Autodesk Inventor part; units mm, degrees
ref_plane "YZ Plane" through (0, 0, 0) normal (1, 0, 0) x (0, 1, 0)
ref_plane "XZ Plane" through (0, 0, 0) normal (0, 1, 0) x (-1, 0, 0)
ref_plane "XY Plane" through (0, 0, 0) normal (0, 0, 1) x (1, 0, 0)
sketch "Sketch1" plane through (0, 0, 0) normal (0, 0, 1) x (1, 0, 0)
  circle A0 centre (0, 0) radius 4.714
extrude "Extrusion1" add sketch "Sketch1" along normal blind 4.7625
fillet "Fillet1" radius 3.175 1 edges at (-4.714, 0, 0)
fillet "Fillet2" radius 0.3175 1 edges at (-4.714, 0, 4.7625)
sketch "Sketch2" plane through (0, 0, 4.7625) normal (0, 0, 1) x (1, 0, 0)
  circle A0 centre (0, 0) radius 1.539
  circle A1 centre (0, 0) radius 2.159
  dimension "d4" = 4.318
extrude "Extrusion2" add sketch "Sketch2" along normal blind 27.94 contours A0 | A1
thread "Thread1"
properties part number "Bolt"
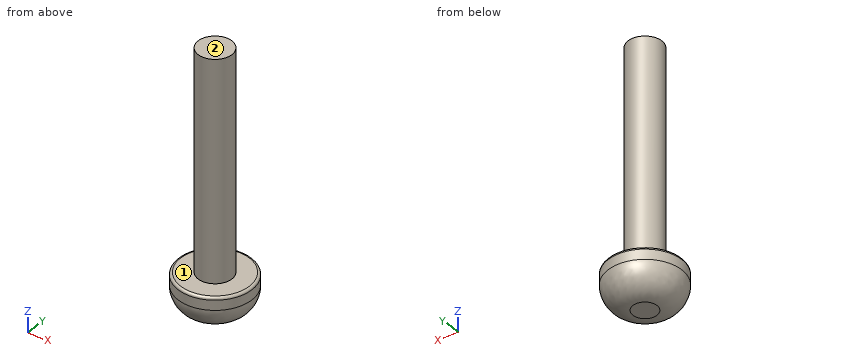
Could you check a few things on this model? Use its own coordinates, in mm. Face numbers are marked on the shaded views. A direction names the side the tool comes from. Round coordinates to 2 decimals unless told otherwise and drop trailing zeros. Write each loop counter-clockwise with the first axis right and the second up, starting at its lowest first coordinate (ties: lowest second). Pieces come first, ordered by that corner, then holes. Notation, with made-up numbers: (73, 71.25) - (115, 71.25) arc R21 cw to (115, 75.25) - close; hole circle Ø11 at (-38, 15.25). An arc over 180 degrees is marked (long way). Use a Markdown table: item, result.
Q1. I want a section at B-B (z = 4). List the corners of the cut face in (x, y) for me.
Output values:
| item | result |
|---|---|
| outline | circle Ø9.43 at (0, 0) |
Q2. For pin 1 (1 mm diameter, centred on x = 0.5, z = 19, fed in from +Y); pin 2 (4 mm diameter, centred on x = 3, z = 26, fed in from -Y); pin 3 (1.5 mm diameter, centred on y = -3, z = 6, fed in from +X), each with a flat end and sliding along its axis, tell me the tip position at first contact or that it passes through.
Output values:
| item | result |
|---|---|
| pin 1 | y = 2.16 |
| pin 2 | y = -1.91 |
| pin 3 | through |
Q3. I want a section at A-A (z = 11). List the corners of the cut face in (x, y) for me, plus the area to 3 significant figures.
Output values:
| item | result |
|---|---|
| outline | circle Ø4.32 at (0, 0) |
| area | 14.6 mm2 |
Q4. For the marked faces 1 and 2, which set-ups out of +Z, -Z, +X, -X, +Y, -Y let a thin tool reach every point of the face, with its end or its side?
Output values:
| item | result |
|---|---|
| face 1 | +Z |
| face 2 | +Z, +X, -X, +Y, -Y |
Q5. Please list where these lines run through material, in increasing order: L1, parallel to Z at x = -3, y = 3; L2, parallel to Y at x = -0.75, z = 20.5; L3, parallel to Z at x = -1.25, y = 1.5.
Output values:
| item | result |
|---|---|
| L1 | 1.51 to 4.76 |
| L2 | -2.02 to 2.02 |
| L3 | 0.03 to 32.7 |
